Work out the finished part from the listing and answer in its coordinate system (mm). A direction names the side the tool comes from. Round coordinates to 2 decimals unless told otherwise and drop trailing zeros. Write each loop counter-clockwise with the first axis right and the second up, starting at its lowest first coordinate (ties: lowest second). Pieces come first, ordered by that corner, then holes.
Autodesk Fusion 360 part; units mm, degrees
sketch "Sketch1" plane through (0, 0, 0) normal (0, 1, 0) x (1, 0, 0)
  line L0 (0, 0) -> (150, 0)
  line L1 (150, 0) -> (150, 150)
  line L2 (150, 150) -> (0, 150)
  line L3 (0, 150) -> (0, 0)
  line L4 (0, 0) -> (134.62, 0)
  line L5 (134.62, 0) -> (134.62, 31.75)
  circle A0 centre (134.62, 31.75) radius 1.6
  line L6 (134.62, 0) -> (134.62, 106.68)
  circle A1 centre (134.62, 106.68) radius 1.6
  line L7 (0, 0) -> (50.8, 0)
  line L8 (50.8, 0) -> (50.8, 106.68)
  line L9 (50.8, 0) -> (50.8, 31.75)
  circle A2 centre (50.8, 106.68) radius 1.6
  circle A3 centre (50.8, 31.75) radius 1.6
  dimension "d1" = 150
  dimension "d2" = 150
  dimension "d3" = 134.62
  dimension "d4" = 31.75
  dimension "d5" = 3.2
  dimension "d6" = 106.68
  dimension "d7" = 3.2
  dimension "d8" = 50.8
  dimension "d9" = 106.68
  dimension "d10" = 31.75
  dimension "d11" = 3.2
  dimension "d12" = 3.2
extrude "Extrude1" add sketch "Sketch1" along normal blind 10
extrude "Extrude2" add 1 faces at (106.3029, 10, -57.1038) along direction (0, 1, 0) blind 20
extrude "Extrude3" cut 1 faces at (0, 10, -100) along direction (1, 0, 0) blind 35.42
extrude "Extrude4" cut 1 faces at (111.8067, 10, -150) along direction (0, 0, 1) blind 10.17
extrude "Extrude5" add 1 faces at (35.42, 10, -93.22) along direction (-1, 0, 0) blind 5
extrude "Extrude6" add 1 faces at (150, 10, -46.61) along direction (1, 0, 0) blind 5
sketch "Sketch2" plane through (0, 30, 0) normal (0, 1, 0) x (-1, 0, 0)
  circle A0 centre (-50.8, -106.68) radius 1.6
  circle A1 centre (-134.62, -31.75) radius 1.6
  circle A2 centre (-50.8, -31.75) radius 1.6
  circle A3 centre (-134.62, -106.68) radius 1.6
  line L0 (-155, -139.83) -> (-30.42, -139.83)
  line L1 (-30.42, -139.83) -> (-30.42, 0)
  line L2 (-30.42, 0) -> (-155, 0)
  line L3 (-155, 0) -> (-155, -139.83)
  line L4 (-30.42, -139.83) -> (-30.42, -129.83)
  line L5 (-155, 0) -> (-145, 0)
  line L6 (-40.42, -129.83) -> (-145, -129.83)
  line L7 (-145, -129.83) -> (-145, -10)
  line L8 (-145, -10) -> (-40.42, -10)
  line L9 (-40.42, -10) -> (-40.42, -129.83)
  dimension "d26" = 10
  dimension "d27" = 10
extrude "Extrude7" add sketch "Sketch2" along normal blind 30 contours L0 L1 L2 L3 L4 L5
sketch "Sketch3" plane through (0, 0, -139.83) normal (0, 0, -1) x (-1, 0, 0)
  line L0 (-155, 60) -> (-155, 0)
  line L1 (-155, 0) -> (-30.42, 0)
  line L2 (-30.42, 0) -> (-30.42, 60)
  line L3 (-30.42, 60) -> (-155, 60)
  line L4 (-155, 60) -> (-155, 55)
  line L5 (-155, 55) -> (-143, 55)
  line L6 (-30.42, 60) -> (-30.42, 55)
  line L7 (-30.42, 55) -> (-42.42, 55)
  line L8 (-42.42, 55) -> (-42.42, 45)
  line L9 (-143, 55) -> (-42.42, 55)
  line L10 (-42.42, 55) -> (-42.42, 45)
  line L11 (-42.42, 45) -> (-143, 45)
  line L12 (-143, 45) -> (-143, 55)
  dimension "d30" = 12
  dimension "d31" = 12
extrude "Extrude8" cut sketch "Sketch3" against normal blind 200 contours L8 L9 L10 L11 L12
Q1. Find section B-B (x = 50.8). Determine the outline of the cut face in (y, z), plus the area to 3 significant figures.
Q2. Find the intervals of material crossed by L1, parallel to X at y = 20, z = -31.75; L2, parallel to Z at x = 134.62, y = 18; L3, parallel to X at y = 54, z = -99.5, in increasing order.
Q3. Find section D-D (z = -106.68). Determine the outline of the cut face in (x, y), plus the area to 3 significant figures.
Q4. Given pin 1 (1.5 mm diameter, centred on x = 135, z = -63.5, fed in from +Y), flat-ended and moving along its own axis, determine where the tip first touches the part or whether it passes through.
Q5. The mould has two halves that part along Y. Classify faces 1 (the face through (30.42, 30, -71)), 2 (the face through (92, 45, -5)), 3 (the face through (92, 0, -69)): +Y half, -Y half, draft (parallel to the pull), parting line (faces both ways), or undercut.
Q6. Find section C-C (z = -69.5). Determine the outline of the cut face in (x, y).
Q7. Find section A-A (y = 43). Determine the outline of the cut face in (x, z).
Q8. A tool of negligible diameter and unlimited length cuts with its end or side. For faces 4 (the face through (40.42, 45, -69)), 5 (the face through (92, 30, 0)), 6 (the face through (42.42, 50, -135)), from which of +Z, -Z, +X, -X, +Y, -Y can it reach the whole face along a straight path? Write none if from no direction.
Report:
1. outline: (0, -139.83) - (45, -139.83) - (45, -129.83) - (30, -129.83) - (30, -108.28) - (0, -108.28) - close; (0, -105.08) - (30, -105.08) - (30, -33.35) - (0, -33.35) - close; (0, -30.15) - (30, -30.15) - (30, -10) - (45, -10) - (45, 0) - (0, 0) - close; (55, -139.83) - (60, -139.83) - (60, -129.83) - (55, -129.83) - close; (55, -10) - (60, -10) - (60, 0) - (55, 0) - close
1. area: 4,400 mm2
2. L1: x = 30.42 to 49.2, 52.4 to 133.02, 136.22 to 155
2. L2: z = -139.83 to -108.28, -105.08 to -33.35, -30.15 to 0
2. L3: x = 30.42 to 40.42, 145 to 155
3. outline: (30.42, 0) - (49.2, 0) - (49.2, 30) - (40.42, 30) - (40.42, 60) - (30.42, 60) - close; (52.4, 0) - (133.02, 0) - (133.02, 30) - (52.4, 30) - close; (136.22, 0) - (155, 0) - (155, 60) - (145, 60) - (145, 30) - (136.22, 30) - close
3. area: 4,150 mm2
4. pin 1: stops at y = 30
5. face 1: draft
5. face 2: undercut
5. face 3: -Y half
6. outline: (30.42, 0) - (155, 0) - (155, 60) - (145, 60) - (145, 30) - (40.42, 30) - (40.42, 60) - (30.42, 60) - close
7. outline: (30.42, -139.83) - (155, -139.83) - (155, 0) - (30.42, 0) - close; hole (40.42, -129.83) - (145, -129.83) - (145, -10) - (40.42, -10) - close
8. face 4: +Y
8. face 5: +Z, +X, -X, +Y, -Y
8. face 6: +Z, -Z
